Here's how the part is built. I have some questions about the finished solid (model axes, mm). Face numbers are marked on the shaded views. Coordinates: 2 decimals unless noted, no trailing zeros. Write each loop counter-clockwise with the first axis right and the second up, starting at its lowest first coordinate (ties: lowest second). Pieces come first, ordered by that corner, then holes. Notation, with made-up numbers: M -29,77.5 L -15,77.5 A14 ccw -15,90.5 Z; hole C 43,79.5 d11. An arc over 180 degrees is marked long. Use a Markdown table: item, result.
```python
from build123d import *

# Parameters (mm, degrees)
F1_DEPTH = 6.35
F2_SIZE  = 18.034


with BuildPart() as f1:
    # F0 (on Front) → F1 (new body, symmetric)
    with BuildSketch(Plane.XZ):
        with BuildLine():
            Line((-45.212, -50.038), (45.212, -50.038))
            Line((45.212, -50.038), (45.212, -62.484))
            Line((45.212, -62.484), (101.346, -62.484))
            Line((101.346, -62.484), (101.346, -28.702))
            Line((101.346, -28.702), (83.07388, -28.702))
            Line((83.07388, -28.702), (83.07388, -9.652))
            Line((83.07388, -9.652), (101.346, -9.652))
            Line((101.346, -9.652), (101.346, 0))
            ThreePointArc((101.346, 0), (98.064572, 8.519419), (89.916, 12.63634))
            Line((89.916, 12.63634), (70.104, 14.627521))
            ThreePointArc((70.104, 14.627521), (53.106495, 21.700368), (42.891581, 37.01689))
            ThreePointArc((42.891581, 37.01689), (36.010992, 46.794292), (24.65913, 50.546))
            Line((24.65913, 50.546), (12.951732, 50.546))
            Line((12.951732, 50.546), (6.35, 25.908))
            Line((6.35, 25.908), (-6.35, 25.908))
            Line((-6.35, 25.908), (-12.951732, 50.546))
            Line((-12.951732, 50.546), (-24.65913, 50.546))
            ThreePointArc((-24.65913, 50.546), (-36.010992, 46.794292), (-42.891581, 37.01689))
            ThreePointArc((-42.891581, 37.01689), (-53.106495, 21.700368), (-70.104, 14.627521))
            Line((-70.104, 14.627521), (-89.916, 12.63634))
            ThreePointArc((-89.916, 12.63634), (-98.064572, 8.519419), (-101.346, 0))
            Line((-101.346, 0), (-101.346, -9.652))
            Line((-101.346, -9.652), (-83.07388, -9.652))
            Line((-83.07388, -9.652), (-83.07388, -28.702))
            Line((-83.07388, -28.702), (-101.346, -28.702))
            Line((-101.346, -28.702), (-101.346, -62.484))
            Line((-101.346, -62.484), (-45.212, -62.484))
            Line((-45.212, -62.484), (-45.212, -50.038))
        make_face()
        with BuildLine():
            ThreePointArc((-39.029952, -21.325139), (-50.915473, -13.092182), (-41.32179, -2.275139))
            Line((-41.32179, -2.275139), (30.210615, -2.275139))
            ThreePointArc((30.210615, -2.275139), (34.418121, -13.932974), (24.470048, -21.325139))
            Line((24.470048, -21.325139), (-39.029952, -21.325139))
        make_face(mode=Mode.SUBTRACT)
    extrude(amount=F1_DEPTH, both=True)

    # F2
    f2_edges = [f1.edges().sort_by_distance(p)[0] for p in [
        (-101.346, 0, -62.484),
        (101.346, 0, -62.484),
    ]]
    chamfer(f2_edges, length=F2_SIZE)


solid = f1.part
```
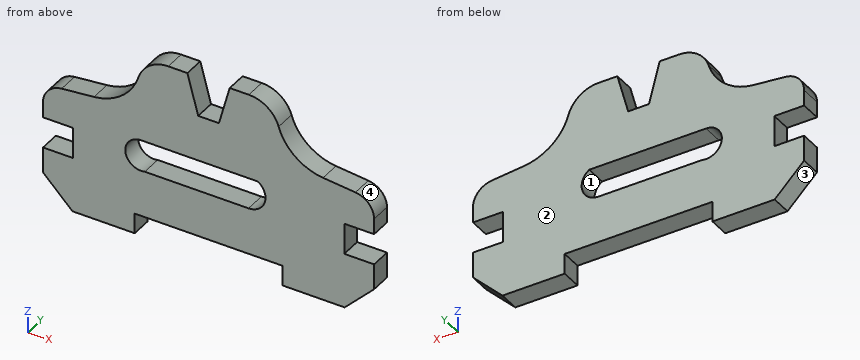
1. I need wall thicknesses on probe 1 along Z at (x, y) = (-22, -3); probe 2 along Z at (x, y) = (0.5, 2.25); probe 3 along X at (y, z) = (-0.5, 36). Which ranges of each line are inside material? Lowest first, please.
Answers follow:
| item | result |
|---|---|
| probe 1 | z = -50.04 to -21.33, -2.28 to 50.55 |
| probe 2 | z = -50.04 to -21.33, -2.28 to 25.91 |
| probe 3 | x = -43.22 to -9.05, 9.05 to 43.22 |
2. Suppose I cut it at A-A on x = -3. Write out the boundary of the cut face in (y, z), and give its area (3 significant figures).
Answers follow:
| item | result |
|---|---|
| outline | M -6.35,-50.04 L 6.35,-50.04 L 6.35,-21.33 L -6.35,-21.33 Z; M -6.35,-2.28 L 6.35,-2.28 L 6.35,25.91 L -6.35,25.91 Z |
| area | 723 mm2 |
3. Will these pins go through, and if not, where does the flat tip stop? pin 1 Ø6.5 at (y, z) = (-0.5, -23.5) entering from +X; pin 2 Ø6.5 at (x, y) = (-88, -0.5) entering from -Z; pin 3 Ø1 at (y, z) = (-2.5, 29) entering from +X.
Answers follow:
| item | result |
|---|---|
| pin 1 | stops at x = 83.07 |
| pin 2 | stops at z = -61.05 |
| pin 3 | stops at x = 46.93 |
4. Suppose I cut it at D-D on z = 9. Write out the boundary of the cut face in (x, y).
Answers follow:
| item | result |
|---|---|
| outline | M -97.61,-6.35 L 97.61,-6.35 L 97.61,6.35 L -97.61,6.35 Z |
5. We'd pull the mould along Z, two halves only. Please class the marked faces 1, 2, 3 and 4: +Z half, -Z half, draft (parallel to the pull), parting line (faces both ways), or undercut.
Answers follow:
| item | result |
|---|---|
| face 1 | undercut |
| face 2 | draft |
| face 3 | -Z half |
| face 4 | +Z half |
6. Suppose I cut it at C-C on z = 32. Write out the boundary of the cut face in (x, y), and give its area (3 significant figures).
Answers follow:
| item | result |
|---|---|
| outline | M -44.89,-6.35 L -7.98,-6.35 L -7.98,6.35 L -44.89,6.35 Z; M 7.98,-6.35 L 44.89,-6.35 L 44.89,6.35 L 7.98,6.35 Z |
| area | 937 mm2 |
